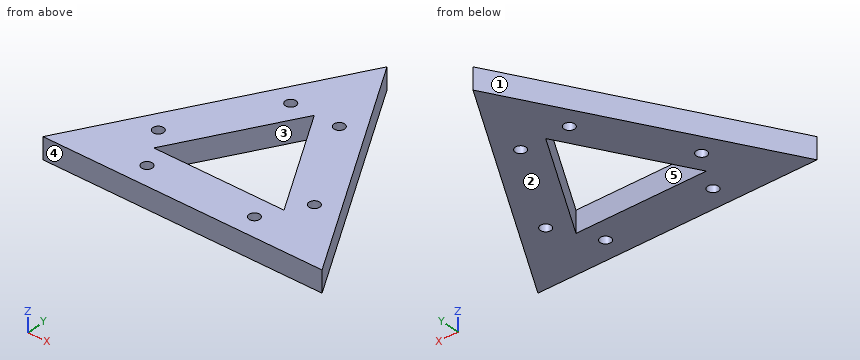
from build123d import *

# Parameters (mm, degrees)
PAD007_DEPTH       = 10
SKETCH012_R        = 2.5
POCKET003_DEPTH    = 354.275599702
POLARPATTERN_COUNT = 3


with BuildPart() as part:
    # Sketch011 → Pad007 (new body)
    with BuildSketch(Plane.XY):
        Polygon((0, 75), (-64.9519052838, -37.5), (64.9519052838, -37.5), align=None)
        Polygon((0, 35), (-30.3108891325, -17.5), (30.3108891325, -17.5), align=None, mode=Mode.SUBTRACT)
    extrude(amount=PAD007_DEPTH)

    # Sketch012 → Pocket003 (cut, through all)
    with BuildSketch(Plane.XY):
        with Locations((11.3156986041, 35.4006350946)):
            Circle(SKETCH012_R)
        with Locations((36.3156986041, -7.9006350946)):
            Circle(SKETCH012_R)
    pocket003 = extrude(amount=POCKET003_DEPTH, mode=Mode.SUBTRACT)

    # PolarPattern: Pocket003 ×3 about axis
    polarpattern_axis = Axis((0, 0, 0), (0, 0, 1))
    for i in range(1, POLARPATTERN_COUNT):
        add(pocket003.rotate(polarpattern_axis, i * 360 / POLARPATTERN_COUNT), mode=Mode.SUBTRACT)


solid = part.part
CAD build for the part. Positions are in the model's coordinates, mm. Face numbers are marked on the shaded views. A direction names the side the tool comes from. Coordinates: 2 decimals unless noted, no trailing zeros. Write each loop counter-clockwise with the first axis right and the second up, starting at its lowest first coordinate (ties: lowest second). Pieces come first, ordered by that corner, then holes. Notation, with made-up numbers: M 14,10 L 57,10 A5 cw 57,14 Z; hole C -1,86 d10. An arc over 180 degrees is marked long. Answer as a JSON object with one key per item and string values. Group by question number.
1) Saw through at D-D (x = -20.5). Write the cut outline in (y, z).
2) Saw through at B-B (z = 4.75). Write the cut outline in (x, y), plus the area to 3 significant figures.
3) Saw through at C-C (y = 18.5). Write the cut outline in (x, z), plus the area to 3 significant figures.
4) Tool access for the marked faces 4 and 5: list every direction of +Z, -Z, +X, -X, +Y, -Y with a clear straight run to the whole face (end or side of a thin tool).
5) Wall check: line 1 (Y direction, x = -10, z = 4.25); line 2 (Y direction, x = -11, z = 2.25); line 3 (X direction, y = 34.5, z = 3.25). Give the ranges that are in metal, low to high. Write a range as from..to.
6) Saw through at A-A (y = -27.5). Write the cut outline in (x, z), plus the area to 3 significant figures.
7) Mould opens along X. For the marked faces 1, 2 and 3 say: +X half, -X half, draft (parallel to the pull), parting line (faces both ways), or undercut.
8) Pin check, flat tips, straight feed: pin 1 Ø6 at (y, z) = (40, 7) entering from -X; pin 2 Ø1 at (x, z) = (29, 3) entering from +Y; pin 3 Ø3 at (x, z) = (-15, 5.5) entering from +Y. Stop position of each tip, or through.
Values follow:
{
 "1": {"outline": "M -37.5,0 L -17.5,0 L -17.5,10 L -37.5,10 Z; M -0.51,0 L 39.49,0 L 39.49,10 L -0.51,10 Z"},
 "2": {"outline": "M -64.95,-37.5 L 64.95,-37.5 L 0,75 Z; hole C -36.32,-7.9 d5; hole M -30.31,-17.5 L 30.31,-17.5 L 0,35 Z; hole C -25,-27.5 d5; hole C -11.32,35.4 d5; hole C 11.32,35.4 d5; hole C 25,-27.5 d5; hole C 36.32,-7.9 d5", "area": "5,600 mm2"},
 "3": {"outline": "M -32.62,0 L -9.53,0 L -9.53,10 L -32.62,10 Z; M 9.53,0 L 32.62,0 L 32.62,10 L 9.53,10 Z", "area": "462 mm2"},
 "4": {"face 4": "+Z, -Z, +X, -X, -Y", "face 5": "+Z, -Z"},
 "5": {"line 1": "y = -37.5..-17.5, 17.68..33.27, 37.53..57.68", "line 2": "y = -37.5..-17.5, 15.95..32.92, 37.88..55.95", "line 3": "x = -23.38..-13.65, -8.98..-0.29, 0.29..8.98, 13.65..23.38"},
 "6": {"outline": "M -59.18,0 L -27.5,0 L -27.5,10 L -59.18,10 Z; M -22.5,0 L 22.5,0 L 22.5,10 L -22.5,10 Z; M 27.5,0 L 59.18,0 L 59.18,10 L 27.5,10 Z", "area": "1,080 mm2"},
 "7": {"face 1": "-X half", "face 2": "draft", "face 3": "undercut"},
 "8": {"pin 1": "stops at x = -21.94", "pin 2": "stops at y = 25.64", "pin 3": "stops at y = 51.62"}
}
